```python
from build123d import *

# Parameters (mm, degrees)
BOSS_EXTRUDE1_DEPTH = 0.4445
SKETCH2_R           = 1.75
CUT_EXTRUDE1_DEPTH  = 204.647238086
FILLET1_R           = 5
SKETCH3_W           = 3
SKETCH3_H           = 6
CUT_EXTRUDE2_DEPTH  = 204.647238086


with BuildPart() as part:
    # Sketch1 → Boss-Extrude1 (new body)
    with BuildSketch(Plane.XY):
        Polygon((144, -21.75), (45, -21.75), (45, -45), (21.75, -45), (21.75, -144), (144, -144), align=None)
    extrude(amount=BOSS_EXTRUDE1_DEPTH)

    # Sketch2 → Cut-Extrude1 (cut, through all)
    with BuildSketch(Plane.XY.offset(0.4445)):
        with Locations((134, -31.75)):
            Circle(SKETCH2_R)
        with Locations((103.375, -62)):
            Circle(SKETCH2_R)
        with BuildLine():
            Line((51, -40.75), (45, -40.75))
            ThreePointArc((45, -40.75), (43.25, -39), (45, -37.25))
            Line((45, -37.25), (51, -37.25))
            ThreePointArc((51, -37.25), (52.75, -39), (51, -40.75))
        make_face()
        with BuildLine():
            Line((31.75, -135.75), (21.75, -135.75))
            ThreePointArc((21.75, -135.75), (20, -134), (21.75, -132.25))
            Line((21.75, -132.25), (31.75, -132.25))
            ThreePointArc((31.75, -132.25), (33.5, -134), (31.75, -135.75))
        make_face()
        with BuildLine():
            Line((101.625, -123.5), (101.625, -120.5))
            ThreePointArc((101.625, -120.5), (103.375, -118.75), (105.125, -120.5))
            Line((105.125, -120.5), (105.125, -123.5))
            ThreePointArc((105.125, -123.5), (103.375, -125.25), (101.625, -123.5))
        make_face()
    extrude(amount=-CUT_EXTRUDE1_DEPTH, mode=Mode.SUBTRACT)

    # Fillet1
    fillet1_edges = [part.edges().sort_by_distance(p)[0] for p in [
        (144, -144, 0.22225),
        (21.75, -144, 0.22225),
        (21.75, -45, 0.22225),
        (45, -21.75, 0.22225),
        (144, -21.75, 0.22225),
    ]]
    fillet(fillet1_edges, radius=FILLET1_R)

    # Sketch3 → Cut-Extrude2 (cut, through all)
    with BuildSketch(Plane(origin=(0, 0, 0), x_dir=(-1, 0, 0), z_dir=(0, 0, -1))):
        with Locations((-41.75, -67)):
            Rectangle(SKETCH3_W, SKETCH3_H)
        with Locations((-54.75, -67)):
            Rectangle(SKETCH3_W, SKETCH3_H)
        with Locations((-41.75, -107)):
            Rectangle(SKETCH3_W, SKETCH3_H)
        with Locations((-54.75, -107)):
            Rectangle(SKETCH3_W, SKETCH3_H)
    extrude(amount=-CUT_EXTRUDE2_DEPTH, mode=Mode.SUBTRACT)


solid = part.part
```
The listing builds one solid part. Answer for the finished solid, in the listing's coordinates (mm). Round coordinates to 2 decimals unless told otherwise and drop trailing zeros. Order: outer loops, then holes, each group sorted by start corner. A loop starts at its lowest first (then second) coordinate and runs counter-clockwise, first axis right, second up. Notation, with made-up numbers: (76.5, 50) -> (113.5, 50) arc R8 ccw to (113.5, 59) -> close; hole circle Ø6 at (-3.5, 60). An arc over 180 degrees is marked (long way). Answer as CSV lines item,"result".
Q1. A cutting plane is placed at B-B on z = 0.15. Give the number of separate pieces and of enclosed holes in the cut face, plus the area to 3 significant figures.
Computed values:
separate pieces,"1"
enclosed holes,"7"
area,"14,200 mm^2"
Q2. For a pull along Y with two mould halves and no side action, classify faces 1 (the cylindrical face through (135.669, -31.224, 0.225)), 2 (the cylindrical face through (103, -63.71, 0.23)), 3 (the flat face through (82, -82, 0.444)), 4 (the cylindrical face through (46.5, -23.18, 0.23)) as +Y half, -Y half, draft (parallel to the pull), parting line (faces both ways), or undercut.
Computed values:
face 1,"undercut"
face 2,"undercut"
face 3,"draft"
face 4,"+Y half"
Q3. Consider line 1 (Y direction, x = 134, z = 0.2); line 2 (X direction, y = -63, z = 0.3); line 3 (Y direction, x = 33, z = 0.35). Determine where each line is inside the solid, lowest interval first. Write a range as from..to.
Computed values:
line 1,"y = -144..-33.5, -30..-21.75"
line 2,"x = 21.75..101.94, 104.81..144"
line 3,"y = -144..-135.22, -132.78..-45"
Q4. A cutting plane is placed at C-C on x = 134. Determine the outline of the cut face in (y, z).
Computed values:
outline,"(-144, 0) -> (-33.5, 0) -> (-33.5, 0.44) -> (-144, 0.44) -> close; (-30, 0) -> (-21.75, 0) -> (-21.75, 0.44) -> (-30, 0.44) -> close"
Q5. A cutting plane is placed at A-A on x = 29. Determine the outline of the cut face in (y, z), plus the area to 3 significant figures.
Computed values:
outline,"(-144, 0) -> (-135.75, 0) -> (-135.75, 0.44) -> (-144, 0.44) -> close; (-132.25, 0) -> (-45, 0) -> (-45, 0.44) -> (-132.25, 0.44) -> close"
area,"42.4 mm^2"
